Design review of the part shown in the three views and the two pictorial views. Dimensions are in mm from the part's minimum x, y and z. A direction names the side the tool comes from. Give positions to 0.01 mm unless a question says otherwise; leave off trailing zeros. Loops run counter-clockwise (first coordinate to the right, second up) from the corner with the lowest first, then second, coordinate; pieces in that order, holes last. Notation, with made-up numbers: (12.25, 13.25) -> (50.25, 13.25) arc R26 ccw to (50.25, 41.25) -> close; hole circle Ø2 at (-22, -14.5). An arc over 180 degrees is marked (long way). One line per question, with ' | ' between items. Start each with the question number.
(1) Draft analysis for pull direction Y (two halves, no side actions). For the marked faces 1, 2 and 3, state which applies: +Y half, -Y half, draft (parallel to the pull), parting line (faces both ways), or undercut.
(2) Consider section D-D (x = 3.5). Write out the cut boundary in (y, z).
(3) Consider section B-B (z = 6.5). Write out the cut boundary in (x, y).
(4) Tool access review of the marked faces 4 and 5: name each direction out of +Z, -Z, +X, -X, +Y, -Y from which nothing blocks a thin tool from reaching the whole face with its end or side.
(5) Wall thickness on probe 1 along X at (y, z) = (7.5, 6); probe 2 along Y at (x, z) = (3, 11.25); probe 3 along Z at (x, y) = (4, 5.5): over which ranges is each line inside the solid? List them lowest first.
(6) Consider section C-C (x = 8.25). Write out the cut boundary in (y, z).
(7) Consider section A-A (y = 3.75). Write out the cut boundary in (x, z), and give its area (3 significant figures).
(8) Insertion check: P1, Ø2, axis at x = 17, y = 4, coming from the -Z side; P2, Ø1.2, axis at x = 12.5, y = 4, coming from the +Z side. Each pin has a flat end and moves straight along its axis. Give the tip position at first contact, or say it passes through.
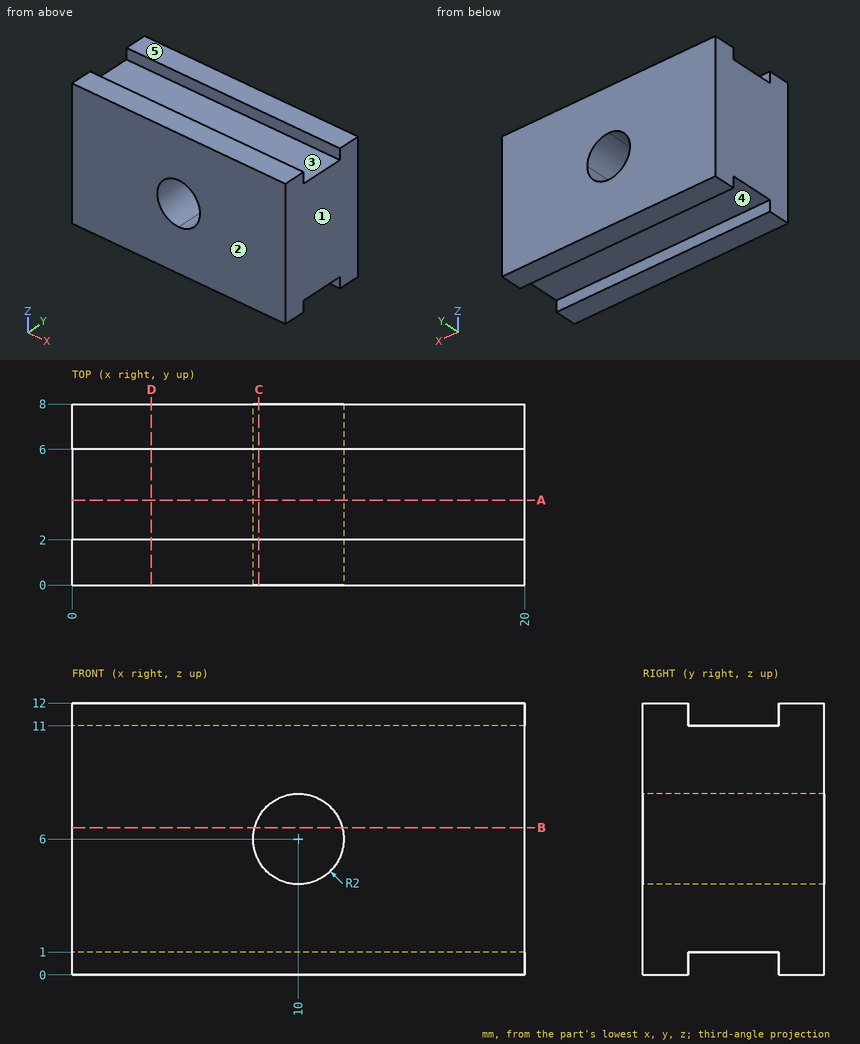
A:
1) face 1: draft | face 2: -Y half | face 3: undercut
2) outline: (0, 0) -> (2, 0) -> (2, 1) -> (6, 1) -> (6, 0) -> (8, 0) -> (8, 12) -> (6, 12) -> (6, 11) -> (2, 11) -> (2, 12) -> (0, 12) -> close
3) outline: (0, 0) -> (8.06, 0) -> (8.06, 8) -> (0, 8) -> close; (11.94, 0) -> (20, 0) -> (20, 8) -> (11.94, 8) -> close
4) face 4: -Z, +X, -X | face 5: +Z, +X, -X, +Y, -Y
5) probe 1: x = 0 to 8, 12 to 20 | probe 2: y = 0 to 2, 6 to 8 | probe 3: z = 1 to 11
6) outline: (0, 0) -> (2, 0) -> (2, 1) -> (6, 1) -> (6, 0) -> (8, 0) -> (8, 5.03) -> (0, 5.03) -> close; (0, 6.97) -> (8, 6.97) -> (8, 12) -> (6, 12) -> (6, 11) -> (2, 11) -> (2, 12) -> (0, 12) -> close
7) outline: (0, 1) -> (20, 1) -> (20, 11) -> (0, 11) -> close; hole circle Ø4 at (10, 6) | area: 187 mm^2
8) P1: stops at z = 1 | P2: stops at z = 11
